Autodesk Inventor part; units mm, degrees
ref_plane "YZ Plane" through (0, 0, 0) normal (1, 0, 0) x (0, 1, 0)
ref_plane "XZ Plane" through (0, 0, 0) normal (0, 1, 0) x (-1, 0, 0)
ref_plane "XY Plane" through (0, 0, 0) normal (0, 0, 1) x (1, 0, 0)
sketch "Sketch1" plane through (0, 0, 0) normal (0, 0, 1) x (1, 0, 0)
  line L0 (0, 0) -> (21.9725, 0)
  line L1 (40.4812, 0) -> (40.4812, 7.9375) construction
  line L2 (40.4812, 7.9375) -> (31.75, 7.9375)
  line L3 (0, 7.9375) -> (0, 6.35)
  line L4 (31.75, 0) -> (31.75, 7.9375) construction
  line L5 (31.75, 9.525) -> (22.225, 9.525)
  line L6 (22.225, 9.525) -> (22.225, 7.9375)
  line L7 (8.7312, 0) -> (8.7312, 17.4625) construction
  line L8 (8.7312, 17.4625) -> (0, 17.4625) construction
  line L9 (0, 17.4625) -> (0, 7.9375) construction
  line L10 (8.7312, 14.2875) -> (9.525, 14.2875) construction
  line L11 (9.525, 14.2875) -> (9.525, 7.9375) construction
  line L12 (9.525, 14.2875) -> (9.525, 27.94) construction
  line L13 (9.525, 27.94) -> (19.05, 27.94) construction
  line L14 (19.05, 27.94) -> (19.05, 7.9375) construction
  line L15 (22.225, 9.525) -> (22.225, 14.2875) construction
  line L16 (22.225, 14.2875) -> (21.4312, 14.2875) construction
  line L17 (21.4312, 14.2875) -> (21.4312, 7.9375) construction
  line L18 (21.4312, 14.2875) -> (21.4312, 17.4625) construction
  line L19 (21.4312, 17.4625) -> (14.2875, 17.4625) construction
  line L20 (14.2875, 17.4625) -> (14.2875, 0) construction
  line L21 (14.2875, 27.94) -> (14.2875, 17.4625) construction
  line L22 (14.1605, 27.94) -> (14.1605, 0) construction
  line L23 (11.9062, 27.94) -> (11.9062, 0) construction
  circle A0 centre (11.9062, 7.5565) radius 2.3813 construction
  line L24 (0, 5.5562) -> (6.2514, 5.5563) construction
  line L25 (0, 6.35) -> (6.2514, 6.35)
  line L26 (6.2514, 6.35) -> (6.2514, 5.5563)
  line L27 (6.2514, 5.5563) -> (6.2514, 0) construction
  line L28 (9.8391, 5.1753) -> (13.9734, 5.1753) construction
  line L29 (0, 3.175) -> (12.7284, 3.175)
  line L30 (6.2514, 5.5563) -> (19.0308, 5.5563)
  line L31 (0, 6.35) -> (0, 0) construction
  circle A1 centre (11.9062, 5.5562) radius 2.3813 construction
  circle A2 centre (11.9062, 5.8103) radius 2.3813 construction
  line L32 (14.2875, 8.1915) -> (9.525, 8.1915) construction
  line L33 (0, 3.175) -> (-5.4674, 3.175)
  line L34 (-5.4674, 3.175) -> (-5.4674, 2.3813)
  line L35 (-5.4674, 2.3813) -> (-10.4458, 2.3812)
  line L36 (-10.4458, 2.3812) -> (-10.4458, 0)
  line L37 (-10.4458, 0) -> (0, 0)
  line L38 (9.8391, 5.1753) -> (7.8389, 3.175) construction
  line L39 (12.7284, 3.175) -> (14.7286, 5.1753)
  line L40 (13.9734, 5.1753) -> (17.083, 0) construction
  line L41 (14.7286, 5.1753) -> (18.8629, 5.1753)
  line L42 (18.8629, 5.1753) -> (21.9725, 0)
  line L43 (19.0308, 5.5563) -> (22.3693, 0)
  line L44 (22.225, 5.5563) -> (31.75, 5.5563) construction
  line L45 (19.0308, 5.5563) -> (22.225, 5.5563) construction
  line L46 (22.225, 7.9375) -> (22.225, 0) construction
  line L47 (31.75, 7.9375) -> (31.75, 9.525)
  line L48 (31.75, 7.9375) -> (22.225, 7.9375) construction
  line L49 (22.225, 7.9375) -> (0, 7.9375)
  line L50 (31.75, 5.5563) -> (40.4812, 5.5563) construction
  line L51 (22.225, 0) -> (40.4812, 0)
  line L52 (22.3693, 0) -> (22.225, 0)
  line L53 (21.9725, 0) -> (22.3693, 0) construction
  line L54 (12.7284, 3.175) -> (40.4812, 3.175) construction
  line L55 (40.4812, 7.9375) -> (101.6, 7.9375)
  line L56 (101.6, 7.9375) -> (101.6, 0)
  line L57 (101.6, 0) -> (40.4812, 0)
  dimension "d0" = 7.9375
  dimension "d1" = 40.4813
  dimension "d2" = 9.525
  dimension "d3" = 8.7312
  dimension "d5" = 22.225
  dimension "d6" = 17.4625
  dimension "d7" = 8.7312
  dimension "d8" = 0.7937
  dimension "d9" = 14.2875
  dimension "d10" = 27.94
  dimension "d11" = 9.525
  dimension "d12" = 0.7937
  dimension "d14" = 7.1437
  dimension "d15" = 17.4625
  dimension "d16" = 0.127
  dimension "d17" = 4.7625
  dimension "d18" = 4.7625
  dimension "d19" = 5.5563
  dimension "d20" = 6.35
  dimension "d22" = 3.175
  dimension "d23" = 4.7625
  dimension "d24" = 4.7625
  dimension "d25" = 4.7625
  dimension "d26" = 0.254
  dimension "d27" = 2.0671
  dimension "d29" = 0.381
  dimension "d30" = 5.4673
  dimension "d31" = 4.9784
  dimension "d32" = 2.3813
  dimension "d33" = 45
  dimension "d34" = 45
  dimension "d35" = 0.0635
  dimension "d36" = 2.0671
  dimension "d37" = 59
  dimension "d38" = 4.1342
  dimension "d39" = 1.5875
  dimension "d40" = 0.3969
  dimension "d41" = 9.525
  dimension "d42" = 14.2875
  dimension "d43" = 61.1187
revolve "Revolution1" add sketch "Sketch1" angle 360 about axis through (0, 0, 0) along (1, 0, 0) contours L37 L36 L35 L34 L33 L29 L39 L41 L42 L0
sketch "Sketch2" plane through (-10.4457, 0, 0) normal (-1, 0, 0) x (0, 0, 1)
  circle A0 centre (0, 0) radius 2.3813
hole "Hole1" at (-10.4457, 0, 0) direction (1, 0, 0) diameter 2.159 depth 5.08 tip angle 118
equation "\"d7\" = d3"
equation "\"d12\" = d8"
equation "\"d15\" = d6"
equation "\"d34\" = d33"
equation "\"d36\" = d27"
equation "\"d38\" = d27 + d36"
equation "\"d42\" = d9"
properties part number "Ball Shift" material "Steel"
Verification items for the finished model (mm, model axes). A direction names the side the tool comes from. Give positions to 0.01 mm unless a question says otherwise; leave off trailing zeros. Loops run counter-clockwise (first coordinate to the right, second up) from the corner with the lowest first, then second, coordinate; pieces in that order, holes last. Notation, with made-up numbers: (89.5, 13.5) - (107.5, 13.5) arc R13 cw to (107.5, 23.5) - close; hole circle Ø5 at (53.25, -10). An arc over 180 degrees is marked (long way). Write item = value, one per line. Start each with the question number.
Q1. Cross-section at A-A, the plane x = -6. Enter the section's corners in (y, z).
Q2. Depth check by flat-ended pin: P1, Ø5, axis at y = -1.5, z = 1, coming from the +X side; P2, Ø2, axis at y = -2, z = 1, coming from the +X side; P3, Ø4, axis at x = -6.5, z = 1, coming from the +Y side (3 decimals). Enter the tip coordinate at first touch or a pass-through.
Q3. Tool access check on faces 1 (the face through (16.82, -0.67, 5.13)), 2 (the face through (-7.99, 1.1, 2.11)). Record the directions out of +Z, -Z, +X, -X, +Y, -Y that give a thin tool (end or side, any length) a straight path to the whole face; none if there is none.
Q4. Mould release check, pull along Y, two halves, no side actions. Record for faces 3 (the face through (-7.87, -1.07, -0.14)), 4 (the face through (21.43, 0.86, -0.27)), 5 (the face through (-4.83, -0.18, -0.04)), 6 (the face through (-10.446, 1, 1)): released by +Y, released by -Y, zero draft, split by the parting line, or undercut.
Q5. Cross-section at C-C, the plane x = 7. Enter the section's corners in (y, z) (3 decimals).
Q6. Cross-section at B-B, the plane x = 16. Enter the section's corners in (y, z).
Q7. Thickness scan on line 1 (Z direction, x = -8.85, y = 0); line 2 (X direction, y = -1, z = 0.5); line 3 (Y direction, x = 12.5, z = 2). Record the ranges inside material, lowest first.
Answer key:
q1.outline = circle Ø4.76 at (0, 0); hole circle Ø2.16 at (0, 0)
q2.P1 = 21.97
q2.P2 = 21.23
q2.P3 = 3.175
q3.face_1 = +X, -X
q3.face_2 = -X
q4.face_3 = undercut
q4.face_4 = split by the parting line
q4.face_5 = undercut
q4.face_6 = zero draft
q5.outline = circle Ø6.35 at (0, 0)
q6.outline = circle Ø10.35 at (0, 0)
q7.line_1 = -2.38 to -1.08, 1.08 to 2.38
q7.line_2 = -10.45 to 21.3
q7.line_3 = -2.47 to 2.47
